Source: CAD feature listing. Evaluate the final solid. Frame: model axes, mm. Face numbers are marked on the shaded views. Give positions to 0.01 mm unless a question says otherwise; leave off trailing zeros. Loops run counter-clockwise (first coordinate to the right, second up) from the corner with the lowest first, then second, coordinate; pieces in that order, holes last. Notation, with made-up numbers: M 50.25,49 L 64.25,49 A19 cw 64.25,58 Z; hole C 3,-19 d10. An arc over 180 degrees is marked long. Answer in a Markdown table with one row per item.
```python
from build123d import *

# Parameters (mm, degrees)
SKETCH1_W           = 19
SKETCH1_H           = 80
BOSS_EXTRUDE1_DEPTH = 35
CUT_EXTRUDE1_DEPTH  = 35
SKETCH3_R           = 5
CUT_EXTRUDE2_DEPTH  = 35
FILLET1_R           = 4


with BuildPart() as part:
    # Sketch1 → Boss-Extrude1 (new body)
    with BuildSketch(Plane(origin=(0, 0, 0), x_dir=(1, 0, 0), z_dir=(0, 1, 0))):
        Rectangle(SKETCH1_W, SKETCH1_H)
    extrude(amount=BOSS_EXTRUDE1_DEPTH)

    # Sketch2 → Cut-Extrude1 (cut)
    with BuildSketch(Plane(origin=(9.5, 0, 0), x_dir=(0, 0, -1), z_dir=(1, 0, 0))):
        with BuildLine():
            ThreePointArc((20.5, 0), (0, 20.5), (-20.5, 0))
            Line((-20.5, 0), (20.5, 0))
        make_face()
        with BuildLine():
            Line((20.5, 0), (-20.5, 0))
            ThreePointArc((-20.5, 0), (0, -20.5), (20.5, 0))
        make_face()
    extrude(amount=-CUT_EXTRUDE1_DEPTH, mode=Mode.SUBTRACT)

    # Sketch3 → Cut-Extrude2 (cut)
    with BuildSketch(Plane.XZ):
        with Locations(Location((0, -30.25, 0), (0, 0, 270))):
            Circle(SKETCH3_R)
        with Locations(Location((0, 30.25, 0), (0, 0, 270))):
            Circle(SKETCH3_R)
    extrude(amount=-CUT_EXTRUDE2_DEPTH, mode=Mode.SUBTRACT)

    # Fillet1
    fillet1_edges = [part.edges().sort_by_distance(p)[0] for p in [
        (9.5, 17.5, 40),
        (-9.5, 17.5, 40),
        (-9.5, 17.5, -40),
        (9.5, 17.5, -40),
    ]]
    fillet(fillet1_edges, radius=FILLET1_R)


solid = part.part
```
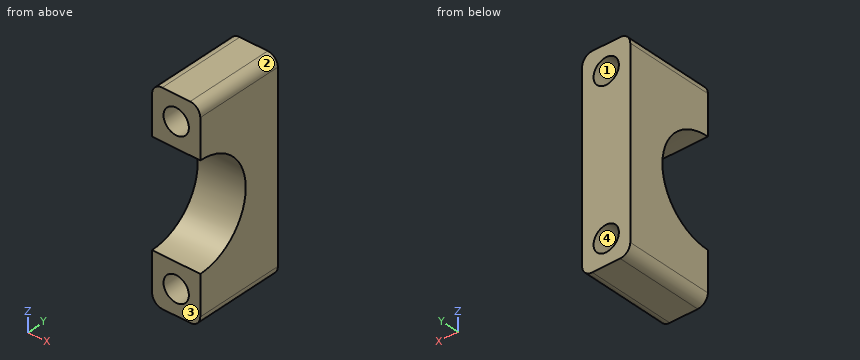
1) Section D-D, the plane y = 23. Return loops of the section in (x, z), then the cut area to 3 significant figures.
Reply:
| item | result |
|---|---|
| outline | M -9.5,-36 A4 ccw -5.5,-40 L 5.5,-40 A4 ccw 9.5,-36 L 9.5,36 A4 ccw 5.5,40 L -5.5,40 A4 ccw -9.5,36 Z; hole C 0,-30.25 d10; hole C 0,30.25 d10 |
| area | 1,350 mm² |
2) Pin query (flat end, axial travel): pin 1 Ø12 at (y, z) = (4.5, 14.5) entering from -X; pin 2 Ø1 at (x, y) = (7, 24) entering from +Z. Return the tip coordinate at first contact, or that it passes through.
Reply:
| item | result |
|---|---|
| pin 1 | stops at x = -9.5 |
| pin 2 | stops at z = 39.87 |
3) Section C-C, the plane z = -30.25. Return loops of the section in (x, y), then the cut area to 3 significant figures.
Reply:
| item | result |
|---|---|
| outline | M -9.5,0 L -5,0 L -5,35 L -9.5,35 Z; M 5,0 L 9.5,0 L 9.5,35 L 5,35 Z |
| area | 315 mm² |
4) Pull-direction query (X, two-part tool) for the marked faces 1, 2, 3 and 4; classes: released by +X, released by -X, zero draft, split by the parting line, or undercut.
Reply:
| item | result |
|---|---|
| face 1 | undercut |
| face 2 | released by +X |
| face 3 | zero draft |
| face 4 | undercut |
5) Material intervals for L1, parallel to X at y = 8.5, z = -30.25; L2, parallel to Z at x = 3.5, y = 6; L3, parallel to Z at x = -2, y = 30.5, sorted ascending.
Reply:
| item | result |
|---|---|
| L1 | x = -9.5 to -5, 5 to 9.5 |
| L2 | z = -40 to -33.82, -26.68 to -19.6, 19.6 to 26.68, 33.82 to 40 |
| L3 | z = -40 to -34.83, -25.67 to 25.67, 34.83 to 40 |
6) Section B-B, the plane y = 10.5. Return loops of the section in (x, z), then the cut area to 3 significant figures.
Reply:
| item | result |
|---|---|
| outline | M -9.5,-36 A4 ccw -5.5,-40 L 5.5,-40 A4 ccw 9.5,-36 L 9.5,-17.61 L -9.5,-17.61 Z; M -9.5,17.61 L 9.5,17.61 L 9.5,36 A4 ccw 5.5,40 L -5.5,40 A4 ccw -9.5,36 Z; hole C 0,-30.25 d10; hole C 0,30.25 d10 |
| area | 680 mm² |
7) Section A-A, the plane x = 0. Return loops of the section in (y, z), then the cut area to 3 significant figures.
Reply:
| item | result |
|---|---|
| outline | M 0,-40 L 35,-40 L 35,-35.25 L 0,-35.25 Z; M 0,-25.25 L 35,-25.25 L 35,25.25 L 0,25.25 L 0,20.5 A20.5 cw 0,-20.5 Z; M 0,35.25 L 35,35.25 L 35,40 L 0,40 Z |
| area | 1,440 mm² |
